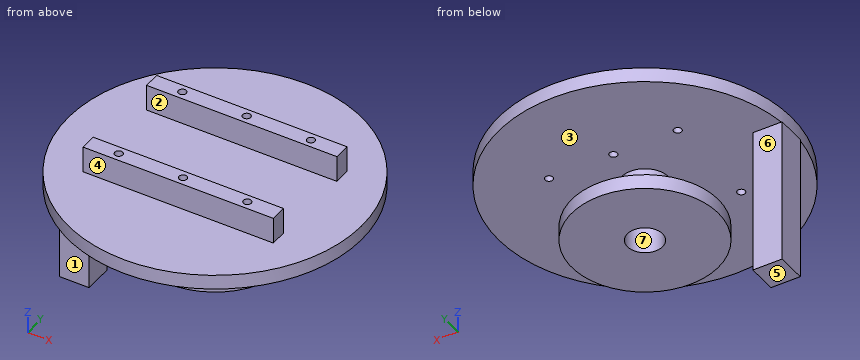
Autodesk Inventor part; units mm, degrees
ref_plane "YZ Plane" through (0, 0, 0) normal (1, 0, 0) x (0, 1, 0)
ref_plane "XZ Plane" through (0, 0, 0) normal (0, 1, 0) x (-1, 0, 0)
ref_plane "XY Plane" through (0, 0, 0) normal (0, 0, 1) x (1, 0, 0)
sketch "Skizze1" plane through (0, 0, 0) normal (0, 0, 1) x (1, 0, 0)
  circle A0 centre (0, 0) radius 50
  dimension "d0" = 100
extrude "Extrusion1" add sketch "Skizze1" along normal blind 5
sketch "Skizze2" plane through (0, 0, 0) normal (0, 0, -1) x (-1, 0, 0)
  circle A0 centre (0, 0) radius 6
  circle A1 centre (0, 0) radius 8
  dimension "d3" = 12
  dimension "d4" = 16
extrude "Extrusion2" add sketch "Skizze2" along normal blind 20
sketch "Skizze3" plane through (0, 0, 0) normal (0, 0, -1) x (-1, 0, 0)
  circle A0 centre (0, 0) radius 50 construction
  line L0 (50, 0) -> (40, 0) construction
  line L1 (40, 0) -> (40, 5) construction
  line L2 (40, 5) -> (50, 5) construction
  line L3 (40, 5) -> (50, 5) construction
  line L4 (50, 5) -> (50, 0) construction
  line L5 (50, 0) -> (50, -5) construction
  line L6 (40, 5) -> (50, 5)
  line L7 (50, 5) -> (50, -5)
  line L8 (50, -5) -> (40, -5)
  line L9 (40, -5) -> (40, 5)
  dimension "d7" = 10
  dimension "d8" = 5
  dimension "d10" = 10
  dimension "d11" = 0
  dimension "d12" = 5
extrude "Extrusion3" add sketch "Skizze3" along normal blind 50
sketch "Skizze4" plane through (0, 0, 5) normal (0, 0, 1) x (1, 0, 0)
  line L0 (-40, 5) -> (-49.7494, 5) construction
  circle A0 centre (0, 0) radius 6 construction
  line L1 (0, 0) -> (32.55, 0) construction
  line L2 (32.55, 0) -> (32.55, -20.3)
  line L3 (0, 0) -> (-32.55, 0) construction
  line L4 (-32.55, 0) -> (-32.55, -20.3) construction
  line L5 (-32.55, 0) -> (-32.55, -20.3) construction
  line L6 (32.55, -20.3) -> (32.55, -14.7) construction
  line L7 (-32.55, -20.3) -> (-32.55, -14.7) construction
  line L8 (-32.55, -20.3) -> (32.55, -20.3)
  line L9 (32.55, -20.3) -> (32.55, -14.7)
  line L10 (32.55, -14.7) -> (-32.55, -14.7)
  line L11 (-32.55, -14.7) -> (-32.55, -20.3)
  dimension "d23" = 32.55
  dimension "d24" = 20.3
  dimension "d25" = 32.55
  dimension "d26" = 20.3
  dimension "d27" = 5.6
  dimension "d28" = 5.6
extrude "Extrusion4" add sketch "Skizze4" along normal blind 9
ref_plane "Arbeitsebene1" through (-32.55, 0, 5) normal (0, 1, 0) x (1, 0, 0)
mirror "Spiegeln1" about plane through (-32.55, 0, 5) normal (0, 1, 0) of "Extrusion4"
sketch "Skizze9" plane through (-32.55, 20.3, 14) normal (0, 0, 1) x (1, 0, 0)
  circle A0 centre (32.5, -2.8) radius 1.35
  circle A1 centre (54.5, -2.8) radius 1.35
  circle A2 centre (10.5, -2.8) radius 1.35
  circle A3 centre (54.5, -2.8) radius 1.4
  circle A4 centre (32.5, -2.8) radius 1.4
  circle A5 centre (10.5, -2.8) radius 1.4
  point P0 (32.55, -20.3)
  dimension "d40" = 2.8
  dimension "d41" = 2.8
  dimension "d42" = 2.8
extrude "Extrusion7" cut sketch "Skizze9" against normal through all contours A0 | A1 | A2
mirror "Spiegeln3" about plane through (-32.55, 0, 5) normal (0, 1, 0) of "Extrusion7"
sketch "Skizze11" plane through (0, 0, -20) normal (0, 0, -1) x (-1, 0, 0)
  circle A0 centre (0, 0) radius 8
  circle A1 centre (0, 0) radius 8
  circle A2 centre (0, 0) radius 25
  dimension "d53" = 16
  dimension "d54" = 50
extrude "Extrusion9" add sketch "Skizze11" against normal blind 5
properties part number "turntable"
Can you work these out from the model? Positions are in its coordinate system, mm. Face numbers are marked on the shaded views. A direction names the side the tool comes from. Round coordinates to 2 decimals unless told otherwise and drop trailing zeros. Write each loop counter-clockwise with the first axis right and the second up, starting at its lowest first coordinate (ties: lowest second). Pieces come first, ordered by that corner, then holes. Notation, with made-up numbers: M 23.25,-27 L 56.25,-27 A18 cw 56.25,-9 Z; hole C 27,43 d3. An arc over 180 degrees is marked long. Use a Markdown table: item, result.
Item 1: I want a section at A-A (z = -8.5). List the corners of the cut face in (x, y) for me.
Found:
| item | result |
|---|---|
| outline | M -50,-5 L -40,-5 L -40,5 L -50,5 Z; C 0,0 d16; hole C 0,0 d12 |
Item 2: I want a section at C-C (y = -17.5). List the corners of the cut face in (x, z) for me.
Found:
| item | result |
|---|---|
| outline | M -46.84,0 L -23.4,0 L -23.4,14 L -32.55,14 L -32.55,5 L -46.84,5 Z; M -20.7,0 L -1.4,0 L -1.4,14 L -20.7,14 Z; M -17.85,-20 L 17.85,-20 L 17.85,-15 L -17.85,-15 Z; M 1.3,0 L 20.6,0 L 20.6,14 L 1.3,14 Z; M 23.3,0 L 46.84,0 L 46.84,5 L 32.55,5 L 32.55,14 L 23.3,14 Z |
Item 3: For pin 1 Ø9.5 at (x, y) = (-2.5, 1.5) entering from -Z; pin 2 Ø1.5 at (x, y) = (-31, -33.5) entering from +Z; pin 3 Ø11 at (x, z) = (-45, -33.5) entering from +Y; pin 4 Ø10 at (x, y) = (-36.5, -4) entering from -Z, each with a flat end and sliding along its axis, tell me the tip position at first contact or that it passes through.
Found:
| item | result |
|---|---|
| pin 1 | stops at z = -20 |
| pin 2 | stops at z = 5 |
| pin 3 | stops at y = 5 |
| pin 4 | stops at z = -50 |
Item 4: I want a section at B-B (x = 21.95). List the corners of the cut face in (y, z) for me, and give its area (3 significant figures).
Found:
| item | result |
|---|---|
| outline | M -44.92,0 L -18.85,0 L -18.85,14 L -20.3,14 L -20.3,5 L -44.92,5 Z; M -16.15,0 L 16.15,0 L 16.15,14 L 14.7,14 L 14.7,5 L -14.7,5 L -14.7,14 L -16.15,14 Z; M -11.97,-20 L 11.97,-20 L 11.97,-15 L -11.97,-15 Z; M 18.85,0 L 44.92,0 L 44.92,5 L 20.3,5 L 20.3,14 L 18.85,14 Z |
| area | 594 mm2 |
Item 5: If I drill on line 1 along X through (y, z) = (-17.5, 9.75); line 2 along Y through (x, z) = (-0.05, 7); line 3 along Y through (x, z) = (-22, 3), over which ranges is the centre line in solid material (lowest first)? Write a range as [from, to].
Found:
| item | result |
|---|---|
| line 1 | x = [-32.55, -23.4], [-20.7, -1.4], [1.3, 20.6], [23.3, 32.55] |
| line 2 | y = [-20.3, -18.85], [-16.15, -14.7], [14.7, 16.15], [18.85, 20.3] |
| line 3 | y = [-44.9, -18.85], [-16.15, 16.15], [18.85, 44.9] |
Item 6: Which directions (+Z, -Z, +X, -X, +Y, -Y) give clear straight access to the entire face, cutting with the end or side of a thin tool? Please do the marked faces 4, 5, 6 and 7.
Found:
| item | result |
|---|---|
| face 4 | +Z, +X, -X, -Y |
| face 5 | -Z, +X, -X, +Y, -Y |
| face 6 | -Z, -X, +Y |
| face 7 | -Z |
Item 7: I want a section at D-D (x = -30). List the corners of the cut face in (y, z) for me.
Found:
| item | result |
|---|---|
| outline | M -40,0 L 40,0 L 40,5 L 20.3,5 L 20.3,14 L 14.7,14 L 14.7,5 L -14.7,5 L -14.7,14 L -20.3,14 L -20.3,5 L -40,5 Z |
Item 8: We'd pull the mould along Y, two halves only. Please class the marked faces 1, 2 and 3: released by +Y, released by -Y, zero draft, split by the parting line, or undercut.
Found:
| item | result |
|---|---|
| face 1 | released by -Y |
| face 2 | undercut |
| face 3 | zero draft |
